from build123d import *

# Parameters (mm, degrees)
F1_DEPTH = 10
F2_R     = 1.6
F3_DEPTH = 23.7
F2_R_2   = 3.5
F4_DEPTH = 8.11


with BuildPart() as f1:
    # F0 (on Top) → F1 (new body)
    with BuildSketch(Plane.XY):
        with BuildLine():
            ThreePointArc((5.55, 3.6633318168), (6.3690658656, 1.9124591499), (6.65, 0))
            ThreePointArc((6.65, 0), (-1.9124591499, -6.3690658656), (-5.55, 3.6633318168))
            ThreePointArc((-5.55, 3.6633318168), (-5.5352837539, 3.6855303232), (-5.5204787204, 3.7076697127))
            add(Edge.make_bspline(
                [(-5.5204787204, 3.7076697127), (-5.3297892382, 4.0203295099), (-5.3804192174, 4.5028316873), (-5.55, 4.8312691983)],
                knots=[0.0105120097, 0.0105120097, 0.0105120097, 0.0105120097, 0.2268448642, 0.2268448642, 0.2268448642, 0.2268448642], degree=3))
            add(Edge.make_bspline(
                [(-5.55, 4.8312691983), (-5.6230599396, 4.9344742738), (-5.6920586566, 5.0230662013), (-5.7572539606, 5.0984029712)],
                knots=[0, 0, 0, 0, 0.1009309198, 0.1009309198, 0.1009309198, 0.1009309198], degree=3))
            add(Edge.make_bspline(
                [(-5.7572539606, 5.0984029712), (-5.8127692495, 5.1426175603), (-6.1763134647, 5.3226921748), (-6.6399504917, 4.8081685915), (-6.9900612717, 4.1319315673)],
                knots=[0.2997379692, 0.2997379692, 0.2997379692, 0.2997379692, 0.350659585, 0.6091967522, 0.6091967522, 0.6091967522, 0.6091967522], degree=3))
            add(Edge.make_bspline(
                [(-6.9900612717, 4.1319315673), (-7.5192866492, 3.1097356941), (-7.9634342646, 1.5245852987), (-7.952605829, 0.2)],
                knots=[0.6091967522, 0.6091967522, 0.6091967522, 0.6091967522, 1, 1, 1, 1], degree=3))
            Line((-7.952605829, 0.2), (-7.952605829, 0))
            Line((-7.952605829, 0), (-7.952605829, -0.2))
            add(Edge.make_bspline(
                [(-7.952605829, -0.2), (-7.7880043421, -5.9189782478), (-3.58719808, -5.5995097942), (-4, -9.65)],
                knots=[0, 0, 0, 0, 10.2433194248, 10.2433194248, 10.2433194248, 10.2433194248], degree=3))
            Line((-4, -9.65), (0, -9.65))
            Line((0, -9.65), (4, -9.65))
            add(Edge.make_bspline(
                [(7.952605829, -0.2), (7.7880043421, -5.9189782478), (3.58719808, -5.5995097942), (4, -9.65)],
                knots=[0, 0, 0, 0, 10.2433194248, 10.2433194248, 10.2433194248, 10.2433194248], degree=3))
            Line((7.952605829, -0.2), (7.952605829, 0))
            Line((7.952605829, 0), (7.952605829, 0.2))
            add(Edge.make_bspline(
                [(6.9900612717, 4.1319315673), (7.5192866492, 3.1097356941), (7.9634342646, 1.5245852987), (7.952605829, 0.2)],
                knots=[0.6091967522, 0.6091967522, 0.6091967522, 0.6091967522, 1, 1, 1, 1], degree=3))
            add(Edge.make_bspline(
                [(5.7572539606, 5.0984029712), (5.8127692495, 5.1426175603), (6.1763134647, 5.3226921748), (6.6399504917, 4.8081685915), (6.9900612717, 4.1319315673)],
                knots=[0.2997379692, 0.2997379692, 0.2997379692, 0.2997379692, 0.350659585, 0.6091967522, 0.6091967522, 0.6091967522, 0.6091967522], degree=3))
            add(Edge.make_bspline(
                [(5.55, 4.8312691983), (5.6230599396, 4.9344742738), (5.6920586566, 5.0230662013), (5.7572539606, 5.0984029712)],
                knots=[0, 0, 0, 0, 0.1009309198, 0.1009309198, 0.1009309198, 0.1009309198], degree=3))
            add(Edge.make_bspline(
                [(5.5204787204, 3.7076697127), (5.3297892382, 4.0203295099), (5.3804192174, 4.5028316873), (5.55, 4.8312691983)],
                knots=[0.0105120097, 0.0105120097, 0.0105120097, 0.0105120097, 0.2268448642, 0.2268448642, 0.2268448642, 0.2268448642], degree=3))
            ThreePointArc((5.5204787204, 3.7076697127), (5.5352837539, 3.6855303232), (5.55, 3.6633318168))
        make_face()
        with BuildLine():
            add(Edge.make_bspline(
                [(5.7572539606, 5.0984029712), (6.726137476, 6.2180013153), (6.8550118896, 4.4101097728), (6.9900612717, 4.1319315673)],
                knots=[0.1009309198, 0.1009309198, 0.1009309198, 0.1009309198, 1.6008902487, 1.6008902487, 1.6008902487, 1.6008902487], degree=3))
            add(Edge.make_bspline(
                [(5.7572539606, 5.0984029712), (5.8127692495, 5.1426175603), (6.1763134647, 5.3226921748), (6.6399504917, 4.8081685915), (6.9900612717, 4.1319315673)],
                knots=[0.2997379692, 0.2997379692, 0.2997379692, 0.2997379692, 0.350659585, 0.6091967522, 0.6091967522, 0.6091967522, 0.6091967522], degree=3))
        make_face()
        with BuildLine():
            add(Edge.make_bspline(
                [(-5.7572539606, 5.0984029712), (-5.8127692495, 5.1426175603), (-6.1763134647, 5.3226921748), (-6.6399504917, 4.8081685915), (-6.9900612717, 4.1319315673)],
                knots=[0.2997379692, 0.2997379692, 0.2997379692, 0.2997379692, 0.350659585, 0.6091967522, 0.6091967522, 0.6091967522, 0.6091967522], degree=3))
            add(Edge.make_bspline(
                [(-5.7572539606, 5.0984029712), (-6.726137476, 6.2180013153), (-6.8550118896, 4.4101097728), (-6.9900612717, 4.1319315673)],
                knots=[0.1009309198, 0.1009309198, 0.1009309198, 0.1009309198, 1.6008902487, 1.6008902487, 1.6008902487, 1.6008902487], degree=3))
        make_face()
    extrude(amount=F1_DEPTH)

    # F2 (on Front) → F3 (cut)
    with BuildSketch(Plane.XZ):
        with Locations((0, 5)):
            Circle(F2_R)
    extrude(amount=F3_DEPTH, mode=Mode.SUBTRACT)

    # F2 (on Front) → F4 (cut)
    with BuildSketch(Plane.XZ):
        with Locations((0, 5)):
            Circle(F2_R_2)
        with Locations((0, 5)):
            Circle(F2_R, mode=Mode.SUBTRACT)
    extrude(amount=F4_DEPTH, mode=Mode.SUBTRACT)


solid = f1.part
CAD build for the part. Positions are in the model's coordinates, mm. A direction names the side the tool comes from. Round coordinates to 2 decimals unless told otherwise and drop trailing zeros. Loops run counter-clockwise (first coordinate to the right, second up) from the corner with the lowest first, then second, coordinate; pieces in that order, holes last.
(1) Two-plate mould, pull along X, no slides. Class faces 3 (the flat face through (0, -7, 0)), 4 (the cylindrical face through (-2.8, -7.1, 2.9)): +X half, -X half, draft (parallel to the pull), parting line (faces both ways), or undercut.
(2) Drop flat-ended pins along their axis: pin 1 (4 mm diameter, centred on x = 0, z = 5, fed in from +Y); pin 2 (1.5 mm diameter, centred on y = -3, z = 5.5, fed in from +X); pin 3 (4 mm diameter, centred on y = -7, z = 6.5, fed in from +X). Give the stop position or say it passes through.
(3) Cut at A-A (x = 0). Give the cut face in (y, z).
(4) Wall check: line 1 along X through (y, z) = (-9.3, 5); line 2 along Z through (x, y) = (0, -7.35); line 3 along X through (y, z) = (0, 8.25). Give the ranges that are in metal, low to high.
(5) Which spindle directions (+Z, -Z, +X, -X, +Y, -Y) get a long thin tool onto all of the face, cutting with end or side? Do faces 1 (the flat face through (0, -7, 10)), 2 (the flat face through (1, -8.11, 3)). Say none if no direction does.
Findings below:
1. face 3: draft
1. face 4: undercut
2. pin 1: stops at y = -8.11
2. pin 2: stops at x = 7.68
2. pin 3: stops at x = 6.23
3. outline: (-9.65, 0) - (-6.65, 0) - (-6.65, 1.5) - (-8.11, 1.5) - (-8.11, 3.4) - (-9.65, 3.4) - close; (-9.65, 6.6) - (-8.11, 6.6) - (-8.11, 8.5) - (-6.65, 8.5) - (-6.65, 10) - (-9.65, 10) - close
4. line 1: x = -3.98 to -1.6, 1.6 to 3.98
4. line 2: z = 0 to 1.5, 8.5 to 10
4. line 3: x = -7.95 to -6.65, 6.65 to 7.95
5. face 1: +Z, +X, -X, +Y, -Y
5. face 2: +Y
